Drawing for the job (mm, zero at the part's lowest x, y, z). Coordinates: 2 decimals unless noted, no trailing zeros. Write each loop counter-clockwise with the first axis right and the second up, starting at its lowest first coordinate (ties: lowest second). Pieces come first, ordered by that corner, then holes. Notation, with made-up numbers: M -38,-29 L -16,-29 A23 ccw -16,-5 Z; hole C 45,8.5 d1. An arc over 180 degrees is marked long. Put each result on its own line as item: value. Start each with the question number.
Q1. Drill centre lines: line 1 along Z through (x, y) = (4, 5.45); line 2 along Z through (x, y) = (2.8, 8) (1 decimal); line 3 along Y through (x, z) = (4.1, 4) (1 decimal). Where is each one in solid material? Low to high.
Q2. Pull direction Y, two halves, no side cores. Call the marked faces 1, 2 and 3: pulls with the +Y half, pulls with the -Y half, needs draft (parallel to the pull), parting line crosses it, or undercut.
Q3. Cut at A-A (y = 5.45). Write the cut outline in (x, z).
Q4. Drop flat-ended pins along their axis: pin 1 (1.5 mm diameter, centred on x = 1, z = 7.5, fed in from +Y); pin 2 (2 mm diameter, centred on x = 2.5, y = 9, fed in from -Z); pin 3 (1 mm diameter, centred on x = 3.5, z = 4, fed in from -Y); pin 4 (3.5 mm diameter, centred on y = 5.45, z = 5, fed in from +X). Give the stop position or say it passes through.
Q5. Cut at B-B (z = 5). Write the cut outline in (x, y).
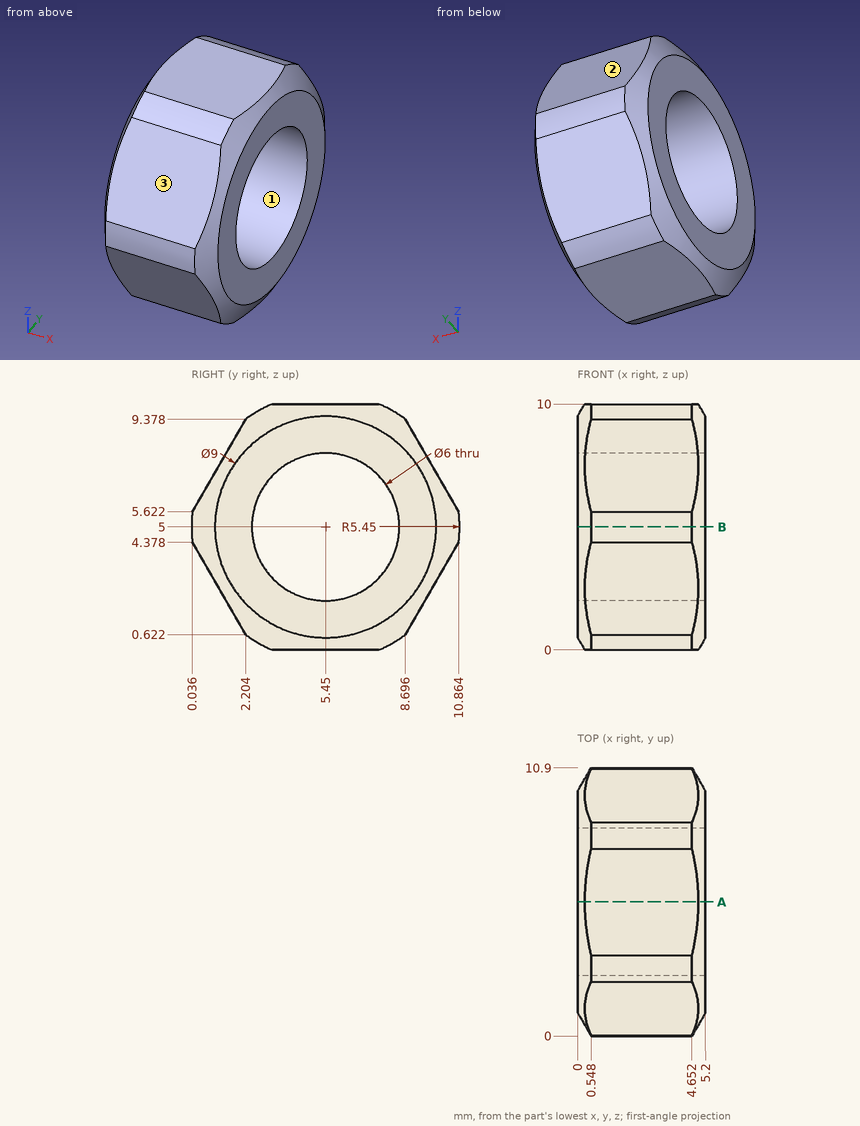
Computed values:
1. line 1: 0 to 2, 8 to 10
1. line 2: 0.2 to 3.4, 6.6 to 9.8
1. line 3: 0.3 to 2.6, 8.3 to 10.6
2. face 1: undercut
2. face 2: pulls with the +Y half
2. face 3: pulls with the -Y half
3. outline: M 0,0.5 L 0.29,0 L 4.91,0 L 5.2,0.5 L 5.2,2 L 0,2 Z; M 0,8 L 5.2,8 L 5.2,9.5 L 4.91,10 L 0.29,10 L 0,9.5 Z
4. pin 1: y = 10.21
4. pin 2: z = 0.18
4. pin 3: y = 0.02
4. pin 4: through
5. outline: M 0,0.95 L 0.55,0 L 4.65,0 L 5.2,0.95 L 5.2,2.45 L 0,2.45 Z; M 0,8.45 L 5.2,8.45 L 5.2,9.95 L 4.65,10.9 L 0.55,10.9 L 0,9.95 Z
